from build123d import *

# Parameters (mm, degrees)
SKETCH1_W           = 374.65
SKETCH1_H           = 406.4
BOSS_EXTRUDE1_DEPTH = 6
SKETCH1_5_W         = 50.8
SKETCH1_5_H         = 50.8
BOSS_EXTRUDE2_DEPTH = 1066.8
SKETCH3_W           = 139.7
SKETCH3_H           = 762
BOSS_EXTRUDE4_DEPTH = 50.8
SKETCH4_W           = 374.65
SKETCH4_H           = 1060.8
BOSS_EXTRUDE5_DEPTH = 10
SKETCH5_W           = 374.65
SKETCH5_H           = 101.6
CUT_EXTRUDE1_DEPTH  = 10
BOSS_EXTRUDE7_REACH = 535.4
SKETCH6_W           = 50.8
SKETCH6_H           = 50.8


with BuildPart() as part:
    # Sketch1 → Boss-Extrude1 (new body)
    with BuildSketch(Plane.XY):
        with Locations((187.325, 203.2)):
            Rectangle(SKETCH1_W, SKETCH1_H)
    extrude(amount=BOSS_EXTRUDE1_DEPTH)

    # Sketch1_5 → Boss-Extrude2 (add)
    with BuildSketch(Plane.XY):
        with Locations((25.4, 381)):
            Rectangle(SKETCH1_5_W, SKETCH1_5_H)
        with Locations((25.4, 25.4)):
            Rectangle(SKETCH1_5_W, SKETCH1_5_H)
        with Locations((349.25, 25.4)):
            Rectangle(SKETCH1_5_W, SKETCH1_5_H)
        with Locations((349.25, 381)):
            Rectangle(SKETCH1_5_W, SKETCH1_5_H)
    extrude(amount=BOSS_EXTRUDE2_DEPTH)

    # Sketch3 → Boss-Extrude4 (add)
    with BuildSketch(Plane.XY.offset(1066.8)):
        with Locations((25.4, 203.2)):
            Rectangle(SKETCH3_W, SKETCH3_H)
        with Locations((349.25, 203.2)):
            Rectangle(SKETCH3_W, SKETCH3_H)
    extrude(amount=BOSS_EXTRUDE4_DEPTH)

    # Sketch4 → Boss-Extrude5 (add)
    with BuildSketch(Plane(origin=(0, 50.8, 0), x_dir=(1, 0, 0), z_dir=(0, 1, 0))):
        with Locations((187.325, -536.4)):
            Rectangle(SKETCH4_W, SKETCH4_H)
    extrude(amount=BOSS_EXTRUDE5_DEPTH)

    # Sketch5 → Cut-Extrude1 (cut)
    with BuildSketch(Plane(origin=(0, 0, 0), x_dir=(-1, 0, 0), z_dir=(0, 0, -1))):
        with Locations((-187.325, 203.2)):
            Rectangle(SKETCH5_W, SKETCH5_H)
    extrude(amount=-CUT_EXTRUDE1_DEPTH, mode=Mode.SUBTRACT)

    # Sketch6 → Boss-Extrude7 (add, up to next)
    with BuildSketch(Plane.XZ.offset(-355.6), mode=Mode.PRIVATE) as boss_extrude7_sk1:
        with Locations((25.4, 31.4)):
            Rectangle(SKETCH6_W, SKETCH6_H)
    boss_extrude7_tool1 = extrude(boss_extrude7_sk1.sketch, amount=BOSS_EXTRUDE7_REACH, mode=Mode.PRIVATE) - part.part
    add(boss_extrude7_tool1.solids().sort_by_distance((25.4, 355.6, 31.4))[0])
    # Sketch6 → Boss-Extrude7 (add, up to next)
    with BuildSketch(Plane.XZ.offset(-355.6), mode=Mode.PRIVATE) as boss_extrude7_sk2:
        with Locations((349.25, 31.4)):
            Rectangle(SKETCH6_W, SKETCH6_H)
    boss_extrude7_tool2 = extrude(boss_extrude7_sk2.sketch, amount=BOSS_EXTRUDE7_REACH, mode=Mode.PRIVATE) - part.part
    add(boss_extrude7_tool2.solids().sort_by_distance((349.25, 355.6, 31.4))[0])


solid = part.part
For this review, take the finished solid that the model builds, in its own axes (mm). A direction names the side the tool comes from. Give positions to 0.01 mm unless a question says otherwise; leave off trailing zeros. Loops run counter-clockwise (first coordinate to the right, second up) from the corner with the lowest first, then second, coordinate; pieces in that order, holes last. Notation, with made-up numbers: (-17.75, 10) - (15.25, 10) arc R23 ccw to (15.25, 39) - close; hole circle Ø2 at (87.5, -38). An arc over 180 degrees is marked (long way). Write each question's results on one line, items separated by ' | '.
(1) Take a section at C-C (y = 235). Give the boundary of the cut face in (x, z).
Conclusion:
outline: (-44.45, 1066.8) - (95.25, 1066.8) - (95.25, 1117.6) - (-44.45, 1117.6) - close; (0, 6) - (50.8, 6) - (50.8, 56.8) - (0, 56.8) - close; (279.4, 1066.8) - (419.1, 1066.8) - (419.1, 1117.6) - (279.4, 1117.6) - close; (323.85, 6) - (374.65, 6) - (374.65, 56.8) - (323.85, 56.8) - close
(2) For line 1 along Z through (x, y) = (280, 12); line 2 along Y through (x, z) = (337, 271.5); line 3 along X through (y, z) = (356, 223), list the stretches that pass through material, from the lowest coordinate up.
Conclusion:
line 1: 0 to 6, 1066.8 to 1117.6 | line 2: 0 to 60.8, 355.6 to 406.4 | line 3: 0 to 50.8, 323.85 to 374.65
(3) Take a section at B-B (z = 576). Give the boundary of the cut face in (x, y), then the cut area to 3 significant figures.
Conclusion:
outline: (0, 0) - (50.8, 0) - (50.8, 50.8) - (323.85, 50.8) - (323.85, 0) - (374.65, 0) - (374.65, 60.8) - (0, 60.8) - close; (0, 355.6) - (50.8, 355.6) - (50.8, 406.4) - (0, 406.4) - close; (323.85, 355.6) - (374.65, 355.6) - (374.65, 406.4) - (323.85, 406.4) - close | area: 14,100 mm^2
(4) Take a section at A-A (x = 196.5). Give the boundary of the cut face in (y, z), then the cut area to 3 significant figures.
Conclusion:
outline: (0, 0) - (152.4, 0) - (152.4, 6) - (60.8, 6) - (60.8, 1066.8) - (50.8, 1066.8) - (50.8, 6) - (0, 6) - close; (254, 0) - (406.4, 0) - (406.4, 6) - (254, 6) - close | area: 12,400 mm^2
(5) For pin 1 Ø12 at (x, z) = (116.5, 701) entering from +Y; pin 2 Ø8 at (y, z) = (408.5, 643.5) entering from -X; pin 3 Ø8 at (x, y) = (212, 388) entering from +Z, all flat-tipped, find the tip position at first contact; note any pin that passes through.
Conclusion:
pin 1: y = 60.8 | pin 2: x = 0 | pin 3: z = 6
(6) For faces 1 (the flat face through (25, 210, 56.8)), 2 (the flat face through (95.25, 198, 1092)), 3 (the flat face through (323.85, 362, 455)), 4 (the flat face through (50.8, 25, 529)), list the 3-axis set-ups (+Z, -Z, +X, -X, +Y, -Y) from which the entire face can be reached by the end or side of a thin tool; tool diameter is ignored.
Conclusion:
face 1: +X, -X | face 2: +Z, +Y, -Y | face 3: +Y | face 4: -Y
(7) Draft analysis for pull direction Y (two halves, no side actions). For faces 5 (the flat face through (419.1, 198, 1092)), 6 (the flat face through (349, 355.6, 555)), 7 (the flat face through (48, 0, 531)), 8 (the flat face through (48, 406.4, 531)), state which applies: +Y half, -Y half, draft (parallel to the pull), parting line (faces both ways), or undercut.
Conclusion:
face 5: draft | face 6: undercut | face 7: -Y half | face 8: +Y half
(8) Take a section at D-D (y = 121.5). Give the boundary of the cut face in (x, z), then the cut area to 3 significant figures.
Conclusion:
outline: (-44.45, 1066.8) - (95.25, 1066.8) - (95.25, 1117.6) - (-44.45, 1117.6) - close; (0, 0) - (374.65, 0) - (374.65, 56.8) - (323.85, 56.8) - (323.85, 6) - (50.8, 6) - (50.8, 56.8) - (0, 56.8) - close; (279.4, 1066.8) - (419.1, 1066.8) - (419.1, 1117.6) - (279.4, 1117.6) - close | area: 21,600 mm^2
